Model file for the job. Use its own axes, mm. Give positions to 0.01 mm unless a question says otherwise; leave off trailing zeros. Loops run counter-clockwise (first coordinate to the right, second up) from the corner with the lowest first, then second, coordinate; pieces in that order, holes last. Notation, with made-up numbers: (-5, 3) - (44, 3) arc R11 ccw to (44, 9) - close; hole circle Ø8 at (48.25, 78.25). An arc over 180 degrees is marked (long way). Use a Markdown table: item, result.
Autodesk Inventor part; units mm, degrees
ref_plane "YZ Plane" through (0, 0, 0) normal (1, 0, 0) x (0, 1, 0)
ref_plane "XZ Plane" through (0, 0, 0) normal (0, 1, 0) x (-1, 0, 0)
ref_plane "XY Plane" through (0, 0, 0) normal (0, 0, 1) x (1, 0, 0)
sketch "Sketch1" plane through (0, 0, 0) normal (0, 0, 1) x (1, 0, 0)
  line L0 (0, 0) -> (150, 0)
  line L1 (150, 0) -> (150, 38.1)
  line L2 (150, 38.1) -> (0, 38.1)
  line L3 (0, 38.1) -> (0, 0)
  line L4 (0, 0) -> (-549.9999, 0)
  line L5 (-549.9999, 0) -> (-549.9999, 38.1)
  line L6 (-549.9999, 38.1) -> (0, 38.1)
  line L7 (0, 38.1) -> (0, 0)
  circle A0 centre (0, 19.05) radius 3.175
  circle A1 centre (137.3, 19.05) radius 3.175
  circle A2 centre (-537.2999, 25.4) radius 3.175
  circle A3 centre (-499.1999, 12.7) radius 3.175
  line L8 (-101.6, 34.29) -> (101.6, 34.29)
  line L9 (101.6, 34.29) -> (101.6, 3.81)
  line L10 (101.6, 3.81) -> (-101.6, 3.81)
  line L11 (-101.6, 3.81) -> (-101.6, 34.29)
  circle A4 centre (-88.9, 27.94) radius 1.5875
  circle A5 centre (-88.9, 10.16) radius 1.5875
  circle A6 centre (-25.4, 10.16) radius 1.5875
  circle A7 centre (-25.4, 27.94) radius 1.5875
  circle A8 centre (25.4, 27.94) radius 1.5875
  circle A9 centre (25.4, 10.16) radius 1.5875
  circle A10 centre (88.9, 10.16) radius 1.5875
  circle A11 centre (88.9, 27.94) radius 1.5875
  point P0 (150, 19.05)
  point P1 (-101.6, 19.05)
  point P2 (0, 15.875)
  point P3 (0, 22.225)
  dimension "d0" = 150
  dimension "d1" = 38.1
  dimension "d2" = 38.1
  dimension "d3" = 549.9999
  dimension "d4" = 6.35
  dimension "d5" = 6.35
  dimension "d6" = 6.35
  dimension "d7" = 6.35
  dimension "d8" = 12.7
  dimension "d9" = 12.7
  dimension "d10" = 12.7
  dimension "d11" = 50.8
  dimension "d12" = 19.05
  dimension "d13" = 12.7
  dimension "d14" = 203.2
  dimension "d15" = 3.81
  dimension "d16" = 3.81
  dimension "d17" = 101.6
  dimension "d18" = 3.175
  dimension "d19" = 3.175
  dimension "d20" = 3.175
  dimension "d21" = 3.175
  dimension "d22" = 3.175
  dimension "d23" = 3.175
  dimension "d24" = 3.175
  dimension "d25" = 3.175
  dimension "d26" = 6.35
  dimension "d27" = 6.35
  dimension "d28" = 6.35
  dimension "d29" = 6.35
  dimension "d30" = 6.35
  dimension "d31" = 6.35
  dimension "d32" = 12.7
  dimension "d33" = 12.7
  dimension "d34" = 12.7
  dimension "d35" = 12.7
  dimension "d36" = 25.4
  dimension "d37" = 25.4
  dimension "d38" = 25.4
  dimension "d39" = 25.4
  dimension "d40" = 6.35
  dimension "d41" = 6.35
extrude "Extrusion1" add sketch "Sketch1" along normal blind 3.175 contours L10 L11 L8 L3 A0 | L3 A0 L8 L9 L10
properties part number "arm"
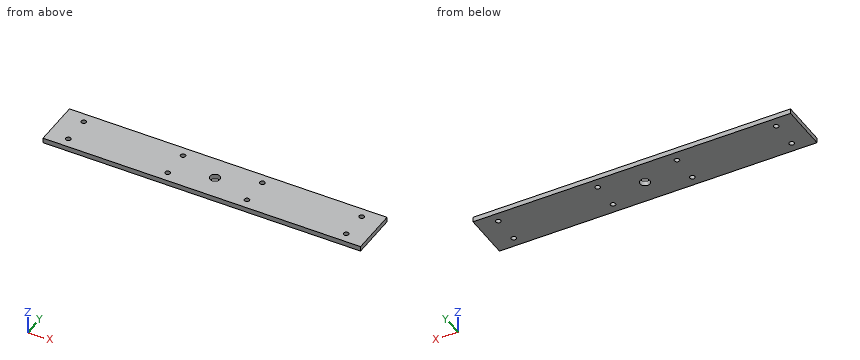
(1) Drill centre lines: probe 1 along Y at (x, z) = (-88.9, 1.85); probe 2 along X at (y, z) = (19, 3.05); probe 3 along X at (y, z) = (27.5, 1.65). Where is each one in solid material? Low to high. Write a range as [from, to].
Computed:
| item | result |
|---|---|
| probe 1 | [3.81, 8.57], [11.75, 26.35], [29.53, 34.29] |
| probe 2 | [-101.6, -3.17], [3.17, 101.6] |
| probe 3 | [-101.6, -90.43], [-87.37, -26.93], [-23.87, 23.87], [26.93, 87.37], [90.43, 101.6] |
(2) Slice it at A-A, the plane x = 0. Write the cut outline in (y, z) (3 decimals).
Computed:
| item | result |
|---|---|
| outline | (3.81, 0) - (15.875, 0) - (15.875, 3.175) - (3.81, 3.175) - close; (22.225, 0) - (34.29, 0) - (34.29, 3.175) - (22.225, 3.175) - close |
(3) Slice it at B-B, the plane z = 2.3. Count the separate pieces of the cut face and the enclosed holes in it, plus the area to 3 significant figures.
Computed:
| item | result |
|---|---|
| separate pieces | 1 |
| enclosed holes | 9 |
| area | 6,100 mm² |
